For this review, take the finished solid that the model builds, in its own axes (mm). Face numbers are marked on the shaded views. Coordinates: 2 decimals unless noted, no trailing zeros. Loops run counter-clockwise (first coordinate to the right, second up) from the corner with the lowest first, then second, coordinate; pieces in that order, holes last. Notation, with made-up numbers: (11, -0.75) - (56, -0.75) arc R32 cw to (56, 27.25) - close; hole circle Ø9 at (62, 88). An arc over 180 degrees is marked (long way). Answer as a JSON object with one key per item and string values. Group by question number.
Item 1: To check wall thickness, follow line 1 (Y direction, x = 23, z = 55); line 2 (X direction, y = -15.5, z = 18); line 3 (X direction, y = -0.75, z = 76.5). State the ranges of each line that lie inside material, in increasing order.
Item 2: We need section B-B (y = -5.5). Give the boundary of the cut face in (x, z), then the cut area to 3 significant figures.
Item 3: We need section C-C (x = 5). Give the boundary of the cut face in (y, z).
Item 4: Mouldability with a two-part tool opening along X and no side actions: class the marked faces 1, 2, 3 and 4 as released by +X, released by -X, zero draft, split by the parting line, or undercut.
Item 5: Clearance check with flat-ended pins moving along their axes: pin 1 (10 mm diameter, centred on x = -43.5, y = -7, fed in from +Z); pin 2 (6 mm diameter, centred on x = 60, z = 49, fed in from -Y); pin 3 (5 mm diameter, centred on x = 29, y = -5, fed in from -Z); pin 4 (6 mm diameter, centred on x = 16.5, z = 15, fed in from +Y). State where each tip first meets the part, or that it passes through.
from build123d import *

# Parameters (mm, degrees)
F1_DEPTH = 19.05
F3_DEPTH = 0.0254


with BuildPart() as f1:
    # F0 (on Front) → F1 (new body)
    with BuildSketch(Plane.XZ):
        with BuildLine():
            ThreePointArc((-24.797919, 5.497566), (0, 25.4), (24.797919, 5.497566))
            Line((24.797919, 5.497566), (80.593235, 17.86709))
            ThreePointArc((80.593235, 17.86709), (0, 82.55), (-80.593235, 17.86709))
            Line((-80.593235, 17.86709), (-24.797919, 5.497566))
        make_face()
    extrude(amount=F1_DEPTH)

    # F2 (on face) → F3 (join)
    with BuildSketch(Plane.XZ.offset(19.05)):
        with BuildLine():
            Line((-0.254, 25.4), (0, 25.4))
            Line((0, 25.4), (0.254, 25.4))
            Line((0.254, 25.4), (0.254, 82.549609))
            ThreePointArc((0.254, 82.549609), (0.127, 82.549902), (0, 82.55))
            ThreePointArc((0, 82.55), (-0.127, 82.549902), (-0.254, 82.549609))
            Line((-0.254, 82.549609), (-0.254, 25.4))
        make_face()
    extrude(amount=F3_DEPTH)


solid = f1.part
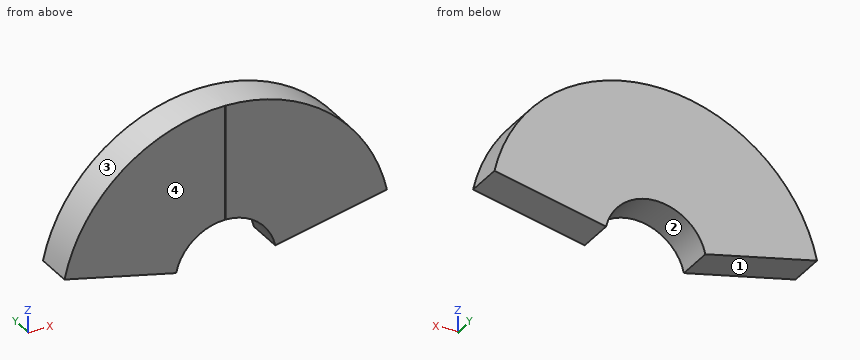
Check sheet entries:
{
 "1": {"line 1": "y = -19.05 to 0", "line 2": "x = -80.56 to -17.92, 17.92 to 80.56", "line 3": "x = -31.02 to 31.02"},
 "2": {"outline": "(-80.59, 17.87) - (-24.8, 5.5) arc R25.4 cw to (24.8, 5.5) - (80.59, 17.87) arc R82.55 ccw to start", "area": "8,340 mm2"},
 "3": {"outline": "(-19.05, 24.9) - (0, 24.9) - (0, 82.4) - (-19.05, 82.4) - close"},
 "4": {"face 1": "released by -X", "face 2": "undercut", "face 3": "split by the parting line", "face 4": "zero draft"},
 "5": {"pin 1": "stops at z = 73.02", "pin 2": "stops at y = -19.05", "pin 3": "stops at z = 5.87", "pin 4": "passes through"}
}
